Source: CAD feature listing. Evaluate the final solid. Frame: model axes, mm. Face numbers are marked on the shaded views. A direction names the side the tool comes from. Give positions to 0.01 mm unless a question says otherwise; leave off trailing zeros. Order: outer loops, then holes, each group sorted by start corner. A loop starts at its lowest first (then second) coordinate and runs counter-clockwise, first axis right, second up. Notation, with made-up numbers: (65.5, 23) -> (89.5, 23) arc R31 ccw to (89.5, 61) -> close; hole circle Ø11 at (-25.5, 51). An arc over 180 degrees is marked (long way). Use CSV: the item, a comma, the result in double quotes.
```python
from build123d import *

# Parameters (mm, degrees)
SKETCH_1_W                = 20
SKETCH_1_H                = 20
SKETCH_1_W_2              = 10
SKETCH_1_H_2              = 10
EXTRUDE_1_DEPTH           = 30
EXTRUDE_1_2_DEPTH         = 20
EXTRUDE_1_2_DEPTH_BACK    = 40
SKETCH_2_W                = 20
SKETCH_2_H                = 20
SKETCH_5_W                = 20
SKETCH_5_H                = 10
CUT_EXTRUDE_1_DEPTH       = 35
SKETCH_6_R                = 1.5
CUT_EXTRUDE_2_DEPTH       = 35
SKETCH_7_W                = 10
SKETCH_7_H                = 10
CUT_EXTRUDE_3_DEPTH       = 35
SKETCH_8_W                = 20
SKETCH_8_H                = 20
CUT_EXTRUDE_4_DEPTH       = 23
SKETCH_10_W               = 20
SKETCH_10_H               = 20
CUT_EXTRUDE_5_DEPTH       = 5
CHAMFER_1_SIZE            = 10
SKETCH_12_W               = 20
SKETCH_12_H               = 15
CUT_EXTRUDE_6_DEPTH       = 5
SKETCH_13_W               = 10
SKETCH_13_H               = 20
CUT_EXTRUDE_7_DEPTH       = 5
SKETCH_14_W               = 40
SKETCH_14_H               = 20
EXTRUDE_4_DEPTH           = 10
SKETCH_15_W               = 10
SKETCH_15_H               = 5
CUT_EXTRUDE_8_DEPTH       = 37
CHAMFER_2_SIZE            = 10
CUT_EXTRUDE_9_DEPTH       = 37
CUT_EXTRUDE_9_DEPTH_BACK  = 10
SKETCH_16_R               = 1.65
SKETCH_18_W               = 40
SKETCH_18_H               = 4
CUT_EXTRUDE_10_DEPTH      = 35
SKETCH_19_W               = 10
SKETCH_19_H               = 8
EXTRUDE_5_DEPTH           = 10
SKETCH_20_R               = 1.5
CUT_EXTRUDE_11_DEPTH      = 30
FILLET_1_R                = 6
SKETCH_21_W               = 10
SKETCH_21_H               = 12
CUT_EXTRUDE_12_DEPTH      = 1
CUT_EXTRUDE_13_DEPTH      = 18
CUT_EXTRUDE_13_DEPTH_BACK = 5
SKETCH_23_W               = 60.486113846
SKETCH_23_H               = 38.876717581
SKETCH_24_W               = 3
SKETCH_24_H               = 3
EXTRUDE_6_DEPTH           = 25
CHAMFER_3_SIZE            = 3
CHAMFER_4_SIZE            = 1
CHAMFER_5_SIZE            = 3


# Some blends are built 0.0001 mm under size
with BuildPart() as part:
    # 草图1 → Extrude 1 (new body)
    with BuildSketch(Plane.XY):
        with Locations((-10, 10)):
            Rectangle(SKETCH_1_W, SKETCH_1_H)
        with Locations((-10, 10)):
            Rectangle(SKETCH_1_W_2, SKETCH_1_H_2, mode=Mode.SUBTRACT)
    extrude(amount=EXTRUDE_1_DEPTH)

    # 草图2 → Extrude 1 2 (add, two sides: drawn at the far end of the back side and taken through both)
    with BuildSketch(Plane(origin=(0, 0, 0), x_dir=(0, 0, -1), z_dir=(1, 0, 0)).offset(-EXTRUDE_1_2_DEPTH_BACK)):
        with Locations((-10, 20)):
            Rectangle(SKETCH_2_W, SKETCH_2_H)
    extrude(amount=EXTRUDE_1_2_DEPTH + EXTRUDE_1_2_DEPTH_BACK)

    # 草图5 → 切除-拉伸1 (cut)
    with BuildSketch(Plane.XY.offset(20)):
        with Locations((-30, 25)):
            Rectangle(SKETCH_5_W, SKETCH_5_H)
        with Locations((10, 25)):
            Rectangle(SKETCH_5_W, SKETCH_5_H)
    extrude(amount=-CUT_EXTRUDE_1_DEPTH, mode=Mode.SUBTRACT)

    # 草图6 → 切除-拉伸2 (cut)
    with BuildSketch(Plane(origin=(0, 30, 0), x_dir=(1, 0, 0), z_dir=(0, 1, 0))):
        with Locations(Location((-21, -10, 0), (0, 0, 311.810314896))):
            Circle(SKETCH_6_R)
        with Locations(Location((1, -10, 0), (0, 0, 228.189685104))):
            Circle(SKETCH_6_R)
    extrude(amount=-CUT_EXTRUDE_2_DEPTH, mode=Mode.SUBTRACT)

    # 草图7 → 切除-拉伸3 (cut)
    with BuildSketch(Plane.XY.offset(30)):
        with Locations((-10, 10)):
            Rectangle(SKETCH_7_W, SKETCH_7_H)
    extrude(amount=-CUT_EXTRUDE_3_DEPTH, mode=Mode.SUBTRACT)

    # 草图8 → 切除-拉伸4 (cut)
    with BuildSketch(Plane(origin=(0, 20, 0), x_dir=(1, 0, 0), z_dir=(0, 1, 0))):
        with Locations((-10, -10)):
            Rectangle(SKETCH_8_W, SKETCH_8_H)
    extrude(amount=CUT_EXTRUDE_4_DEPTH, mode=Mode.SUBTRACT)

    # 草图10 → 切除-拉伸5 (cut)
    with BuildSketch(Plane.XZ.offset(-10)):
        with Locations((-30, 10)):
            Rectangle(SKETCH_10_W, SKETCH_10_H)
        with Locations((10, 10)):
            Rectangle(SKETCH_10_W, SKETCH_10_H)
    extrude(amount=-CUT_EXTRUDE_5_DEPTH, mode=Mode.SUBTRACT)

    # 倒角1
    chamfer_1_edges = [part.edges().sort_by_distance(p)[0] for p in [
        (0, 17.5, 20),
        (-20, 17.5, 20),
    ]]
    chamfer(chamfer_1_edges, length=CHAMFER_1_SIZE - 0.0001)  # a hair under: the kernel refuses the full size

    # 草图12 → 切除-拉伸6 (cut)
    with BuildSketch(Plane.XZ.offset(-15)):
        with Locations((-10, 7.5)):
            Rectangle(SKETCH_12_W, SKETCH_12_H)
    extrude(amount=CUT_EXTRUDE_6_DEPTH, mode=Mode.SUBTRACT)

    # 草图13 → 切除-拉伸7 (cut)
    with BuildSketch(Plane.XZ.offset(-15)):
        with Locations((-35, 10)):
            Rectangle(SKETCH_13_W, SKETCH_13_H)
        with Locations((15, 10)):
            Rectangle(SKETCH_13_W, SKETCH_13_H)
    extrude(amount=-CUT_EXTRUDE_7_DEPTH, mode=Mode.SUBTRACT)

    # 草图14 → 凸台-拉伸4 (add)
    with BuildSketch(Plane.XZ):
        with Locations((-10, 10)):
            Rectangle(SKETCH_14_W, SKETCH_14_H)
    extrude(amount=-EXTRUDE_4_DEPTH)

    # 草图15 → 切除-拉伸8 (cut)
    with BuildSketch(Plane.XY.offset(30)):
        with Locations((-10, 7.5)):
            Rectangle(SKETCH_15_W, SKETCH_15_H)
    extrude(amount=-CUT_EXTRUDE_8_DEPTH, mode=Mode.SUBTRACT)

    # 倒角2
    chamfer_2_edges = [part.edges().sort_by_distance(p)[0] for p in [
        (0, 5, 20),
        (-20, 5, 20),
    ]]
    chamfer(chamfer_2_edges, length=CHAMFER_2_SIZE - 0.0001)  # a hair under: the kernel refuses the full size

    # 草图16 → 切除-拉伸9 (cut, two sides: drawn at the far end of the back side and taken through both)
    with BuildSketch(Plane(origin=(0, 10, 0), x_dir=(1, 0, 0), z_dir=(0, 1, 0)).offset(-CUT_EXTRUDE_9_DEPTH_BACK)):
        with Locations(Location((-21, -10, 0), (0, 0, 90))):
            Circle(SKETCH_16_R)
        with Locations(Location((1, -10, 0), (0, 0, 90))):
            Circle(SKETCH_16_R)
    extrude(amount=CUT_EXTRUDE_9_DEPTH + CUT_EXTRUDE_9_DEPTH_BACK, mode=Mode.SUBTRACT)

    # 草图18 → 切除-拉伸10 (cut)
    with BuildSketch(Plane(origin=(0, 20, 0), x_dir=(1, 0, 0), z_dir=(0, 1, 0))):
        with Locations((-10, -2)):
            Rectangle(SKETCH_18_W, SKETCH_18_H)
    extrude(amount=-CUT_EXTRUDE_10_DEPTH, mode=Mode.SUBTRACT)

    # 草图19 → 凸台-拉伸5 (add)
    with BuildSketch(Plane.XZ):
        with Locations((-10, 20)):
            Rectangle(SKETCH_19_W, SKETCH_19_H)
    extrude(amount=EXTRUDE_5_DEPTH)

    # 草图20 → 切除-拉伸11 (cut)
    with BuildSketch(Plane.ZY.offset(15)):
        with Locations((20, -3)):
            Circle(SKETCH_20_R)
    extrude(amount=-CUT_EXTRUDE_11_DEPTH, mode=Mode.SUBTRACT)

    # 圆角1
    fillet_1_edges = [part.edges().sort_by_distance(p)[0] for p in [
        (-30, 5, 4),
        (10, 5, 4),
        (-30, 17.5, 4),
        (10, 17.5, 4),
    ]]
    fillet(fillet_1_edges, radius=FILLET_1_R)

    # 草图21 → 切除-拉伸12 (cut)
    with BuildSketch(Plane.XZ):
        with Locations((-10, 10)):
            Rectangle(SKETCH_21_W, SKETCH_21_H)
    extrude(amount=-CUT_EXTRUDE_12_DEPTH, mode=Mode.SUBTRACT)

    # 草图23 → 切除-拉伸13 (cut, two sides: drawn at the far end of the back side and taken through both)
    with BuildSketch(Plane.XZ.offset(-CUT_EXTRUDE_13_DEPTH_BACK)):
        with Locations((-10.757338654, 16.810917803)):
            Rectangle(SKETCH_23_W, SKETCH_23_H)
    extrude(amount=CUT_EXTRUDE_13_DEPTH + CUT_EXTRUDE_13_DEPTH_BACK, mode=Mode.SUBTRACT)

    # 草图24 → 凸台-拉伸6 (add)
    with BuildSketch(Plane.XY.offset(30)):
        with Locations((-13.5, 6.5)):
            Rectangle(SKETCH_24_W, SKETCH_24_H)
        with Locations((-6.5, 6.5)):
            Rectangle(SKETCH_24_W, SKETCH_24_H)
    extrude(amount=-EXTRUDE_6_DEPTH)

    # 倒角3
    # the kernel refuses this chamfer: 3 mm, written as the material it adds along each edge
    with BuildSketch(Plane(origin=(-5, 8, 5), x_dir=(0.02749587661058649, 0, -0.9996219169112968), z_dir=(0, -1, 0))) as chamfer_3_piece_1_section:
        Polygon((CHAMFER_3_SIZE * 0.999621916911, -CHAMFER_3_SIZE * 0.0274958766106), (-CHAMFER_3_SIZE * 0.0274958766106, -CHAMFER_3_SIZE * 0.999621916911), (0, 0), align=None)
    chamfer_3_piece_1 = extrude(amount=3, mode=Mode.PRIVATE)
    chamfer_3_piece_1 = split(chamfer_3_piece_1, bisect_by=Plane(origin=(-6.280814641, 6.5, 4), z_dir=(0, 0, 1)), keep=Keep.TOP, mode=Mode.PRIVATE)
    chamfer_3_piece_1 = split(chamfer_3_piece_1, bisect_by=Plane(origin=(-8, 6.5, 4.572987798), z_dir=(1, 0, 0)), keep=Keep.TOP, mode=Mode.PRIVATE)
    add(chamfer_3_piece_1)
    with BuildSketch(Plane(origin=(-15, 8, 5), x_dir=(-0.027495876610586202, 0, -0.9996219169112968), z_dir=(0, -1, 0))) as chamfer_3_piece_2_section:
        Polygon((CHAMFER_3_SIZE * 0.999621916911, CHAMFER_3_SIZE * 0.0274958766106), (-CHAMFER_3_SIZE * 0.0274958766106, CHAMFER_3_SIZE * 0.999621916911), (0, 0), align=None)
    chamfer_3_piece_2 = extrude(amount=3, mode=Mode.PRIVATE)
    chamfer_3_piece_2 = split(chamfer_3_piece_2, bisect_by=Plane(origin=(-13.719185359, 6.5, 4), z_dir=(0, 0, 1)), keep=Keep.TOP, mode=Mode.PRIVATE)
    chamfer_3_piece_2 = split(chamfer_3_piece_2, bisect_by=Plane(origin=(-12, 6.5, 4.572987798), z_dir=(-1, 0, 0)), keep=Keep.TOP, mode=Mode.PRIVATE)
    add(chamfer_3_piece_2)

    # 倒角4
    chamfer_4_edges = [part.edges().sort_by_distance(p)[0] for p in [
        (-12, 8, 17.5),
        (-8, 8, 17.5),
    ]]
    chamfer(chamfer_4_edges, length=CHAMFER_4_SIZE)

    # 倒角5
    chamfer_5_edges = [part.edges().sort_by_distance(p)[0] for p in [
        (0, 12.5, 15),
        (-20, 12.5, 15),
    ]]
    chamfer(chamfer_5_edges, length=CHAMFER_5_SIZE)


solid = part.part
```
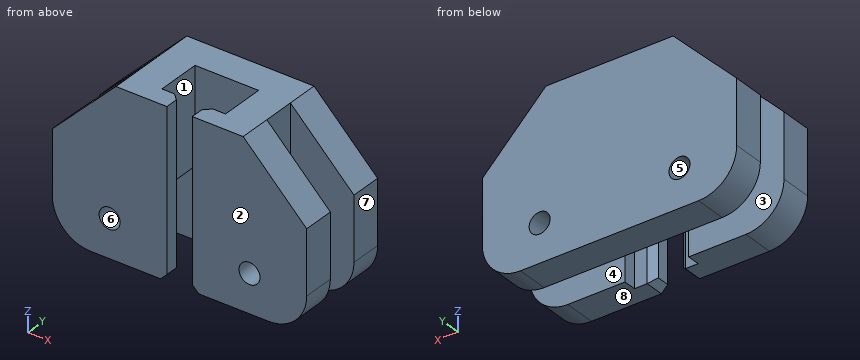
1. Section query D-D on x = 1. Return loops of the section in (y, z), plus the area to 3 significant figures.
Answer below:
outline,"(5, 4) -> (10, 4) -> (10, 8.35) -> (5, 8.35) -> close; (5, 11.65) -> (10, 11.65) -> (10, 29) -> (5, 29) -> close; (15, 4) -> (20, 4) -> (20, 8.35) -> (15, 8.35) -> close; (15, 11.65) -> (20, 11.65) -> (20, 29) -> (15, 29) -> close"
area,"217 mm²"
2. Access query for the marked faces 1, 2, 3 and 4. Directions: +Z, -Z, +X, -X, +Y, -Y. A direction counts if a zero-diameter tool reaches every point of the face in a straight line with its end or side. Return the directions, or none.
Answer below:
face 1,"+Z, -Z"
face 2,"+Z, -Z, +X, -X, -Y"
face 3,"-Z, -X"
face 4,"-Z, +X"
3. Section query B-B on y = 10.75. Return loops of the section in (x, z), plus the area to 3 significant figures.
Answer below:
outline,"(-20, 18) -> (-17, 15) -> (-15, 15) -> (-15, 30) -> (-20, 30) -> close; (-5, 15) -> (-3, 15) -> (0, 18) -> (0, 30) -> (-5, 30) -> close"
area,"141 mm²"
4. Mould query, pull axis X, two halves, no side actions, for the marked faces 5, 6, 7 and 8. Classes: released by +X, released by -X, zero draft, split by the parting line, or undercut.
Answer below:
face 5,"undercut"
face 6,"undercut"
face 7,"released by +X"
face 8,"zero draft"
5. Ray query, line 1 along X through (y, z) = (17, 10); line 2 along X through (y, z) = (14.25, 28); line 3 along X through (y, z) = (8.5, 17.5). Return the intervals inside material, ascending.
Answer below:
line 1,"x = -30 to -22.65, -19.35 to -0.65, 2.65 to 10"
line 2,"x = -20 to -15, -5 to 0"
line 3,"x = -30 to -15, -5 to 10"
6. Pin query (flat end, axial travel): P1, Ø6, axis at y = 10.5, z = 26, coming from the +X side; P2, Ø1.5, axis at y = 15.5, z = 21.5, coming from the +X side; P3, Ø1, axis at x = -16, y = 13, coming from the -Z side. Return the tip coordinate at first contact, or that it passes through.
Answer below:
P1,"stops at x = 6.96"
P2,"stops at x = 9.25"
P3,"stops at z = 15"
7. Section query A-A on y = 8.5. Count the separate pieces of the cut face and the enclosed holes in it, plus the area to 3 significant figures.
Answer below:
separate pieces,"2"
enclosed holes,"2"
area,"647 mm²"
